```python
from build123d import *

# Parameters (mm, degrees)
SKETCH1_W            = 66.5
SKETCH1_H            = 64.5
BOSS_EXTRUDE1_DEPTH  = 25
SKETCH2_W            = 63.5
SKETCH2_H            = 61.5
CUT_EXTRUDE2_DEPTH   = 23.5
SKETCH9_W            = 10
SKETCH9_H            = 5
BOSS_EXTRUDE5_DEPTH  = 5
SKETCH14_R           = 1.5
CUT_EXTRUDE4_DEPTH   = 9
SKETCH17_W           = 10
SKETCH17_H           = 2.5
BOSS_EXTRUDE7_DEPTH  = 5
SKETCH18_R           = 1.5
CUT_EXTRUDE6_DEPTH   = 9
SKETCH19_R           = 1.5
BOSS_EXTRUDE9_DEPTH  = 8
SKETCH22_R           = 1.015
CUT_EXTRUDE7_DEPTH   = 7.5
SKETCH23_W           = 56
SKETCH23_H           = 20
BOSS_EXTRUDE12_DEPTH = 3
SKETCH26_W           = 42
SKETCH26_H           = 20
CUT_EXTRUDE9_DEPTH   = 3
CUT_EXTRUDE12_DEPTH  = 3
CUT_EXTRUDE13_DEPTH  = 3
SKETCH51_W           = 15
SKETCH51_H           = 8
CUT_EXTRUDE14_DEPTH  = 1.5


with BuildPart() as part:
    # Sketch1 → Boss-Extrude1 (new body)
    with BuildSketch(Plane.XY):
        Rectangle(SKETCH1_W, SKETCH1_H)
    extrude(amount=BOSS_EXTRUDE1_DEPTH)

    # Sketch2 → Cut-Extrude2 (cut)
    with BuildSketch(Plane.XY.offset(25)):
        Rectangle(SKETCH2_W, SKETCH2_H)
    extrude(amount=-CUT_EXTRUDE2_DEPTH, mode=Mode.SUBTRACT)

    # Sketch9 → Boss-Extrude5 (add)
    with BuildSketch(Plane.ZY.offset(33.25)):
        with Locations((20, 0)):
            Rectangle(SKETCH9_W, SKETCH9_H)
    extrude(amount=-BOSS_EXTRUDE5_DEPTH)

    # Sketch14 → Cut-Extrude4 (cut)
    with BuildSketch(Plane.XY.offset(25)):
        with Locations((-30.75, 0.228198866)):
            Circle(SKETCH14_R)
    extrude(amount=-CUT_EXTRUDE4_DEPTH, mode=Mode.SUBTRACT)

    # Sketch17 → Boss-Extrude7 (add)
    with BuildSketch(Plane(origin=(33.25, 0, 0), x_dir=(0, 0, -1), z_dir=(1, 0, 0))):
        with Locations((-20, 1.25)):
            Rectangle(SKETCH17_W, SKETCH17_H)
        with Locations((-20, -1.25)):
            Rectangle(SKETCH17_W, SKETCH17_H)
    extrude(amount=-BOSS_EXTRUDE7_DEPTH)

    # Sketch18 → Cut-Extrude6 (cut)
    with BuildSketch(Plane.XY.offset(25)):
        with Locations((30.75, 0)):
            Circle(SKETCH18_R)
    extrude(amount=-CUT_EXTRUDE6_DEPTH, mode=Mode.SUBTRACT)

    # Sketch19 → Boss-Extrude9 (add)
    with BuildSketch(Plane.XY.offset(1.5)):
        with Locations((-20.04, 29.09)):
            Circle(SKETCH19_R)
        with Locations(Location((30.04, 29.09, 0), (0, 0, 180))):
            Circle(SKETCH19_R)
        with Locations(Location((-20.04, -19.09, 0), (0, 0, 180))):
            Circle(SKETCH19_R)
        with Locations((30.04, -18.96)):
            Circle(SKETCH19_R)
    extrude(amount=BOSS_EXTRUDE9_DEPTH)

    # Sketch22 → Cut-Extrude7 (cut)
    with BuildSketch(Plane.XY.offset(9.5)):
        with Locations((-20.04, 29.09)):
            Circle(SKETCH22_R)
        with Locations((30.04, 29.049098521)):
            Circle(SKETCH22_R)
        with Locations((30.04, -18.96)):
            Circle(SKETCH22_R)
        with Locations((-20.04, -19.09)):
            Circle(SKETCH22_R)
    extrude(amount=-CUT_EXTRUDE7_DEPTH, mode=Mode.SUBTRACT)

    # Sketch23 → Boss-Extrude12 (add)
    with BuildSketch(Plane.XY.offset(1.5)):
        with Locations((3.75, 14.75)):
            Rectangle(SKETCH23_W, SKETCH23_H)
    extrude(amount=BOSS_EXTRUDE12_DEPTH)

    # Sketch26 → Cut-Extrude9 (cut)
    with BuildSketch(Plane.XY.offset(4.5)):
        with Locations((4.75, 14.75)):
            Rectangle(SKETCH26_W, SKETCH26_H)
    extrude(amount=-CUT_EXTRUDE9_DEPTH, mode=Mode.SUBTRACT)

    # Sketch45 → Cut-Extrude12 (cut)
    with BuildSketch(Plane(origin=(33.25, 0, 0), x_dir=(0, 0, -1), z_dir=(1, 0, 0))):
        Polygon((-9.814807173, 15.135540206), (-6.214807173, 15.135540206), (-6.214807173, 24.735863123), (-6.214807173, 25.135540206), (-9.814807173, 25.135540206), align=None)
        Polygon((-6.214807173, 4.436476389), (-6.214807173, 13.135540206), (-9.714807173, 13.135540206), (-9.714807173, 3.135540206), (-6.214807173, 3.135540206), align=None)
    extrude(amount=-CUT_EXTRUDE12_DEPTH, mode=Mode.SUBTRACT)

    # Sketch46 → Cut-Extrude13 (cut)
    with BuildSketch(Plane(origin=(0, 32.25, 0), x_dir=(1, 0, 0), z_dir=(0, 1, 0))):
        Polygon((-11.263140916, -11.9), (-11.75, -11.9), (-11.75, -21.9), (-1.75, -21.9), (-1.75, -11.9), align=None)
    extrude(amount=-CUT_EXTRUDE13_DEPTH, mode=Mode.SUBTRACT)

    # Sketch51 → Cut-Extrude14 (cut)
    with BuildSketch(Plane(origin=(0, 32.25, 0), x_dir=(1, 0, 0), z_dir=(0, 1, 0))):
        with Locations((16.75, -15.9)):
            Rectangle(SKETCH51_W, SKETCH51_H)
    extrude(amount=-CUT_EXTRUDE14_DEPTH, mode=Mode.SUBTRACT)


solid = part.part
```
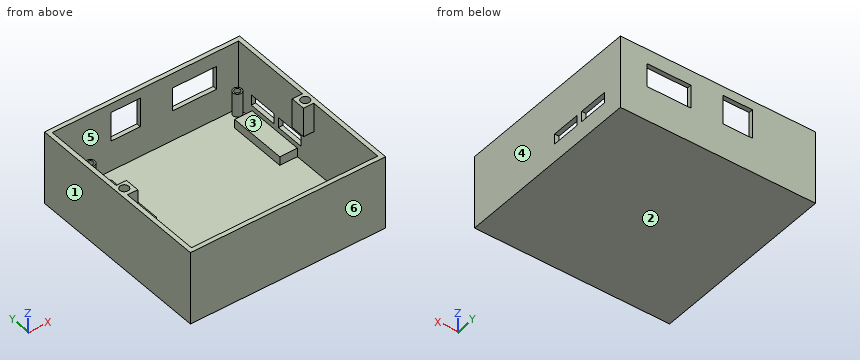
Input: part model. Units: mm. Frame: model coordinates. Face numbers are marked on the shaded views. A direction names the side the tool comes from. Round coordinates to 2 decimals unless told otherwise and drop trailing zeros. Loops run counter-clockwise (first coordinate to the right, second up) from the corner with the lowest first, then second, coordinate; pieces in that order, holes last. Notation, with made-up numbers: (-15, 85.5) - (15, 85.5) arc R24 cw to (15, 101.5) - close; hole circle Ø11 at (32.5, 70.5). An arc over 180 degrees is marked (long way). One line per item, written item: value. Start each with the question number.
(1) Draft query along X for the marked faces 1, 2, 3 and 4. Return one class per face: +X half, -X half, draft (parallel to the pull), parting line (faces both ways), or undercut.
(2) Access query for the marked faces 5 and 6. Directions: +Z, -Z, +X, -X, +Y, -Y. A direction counts if a zero-diameter tool reaches every point of the face in a straight line with its end or side. Return the directions, or none.
(3) Section D-D, the plane z = 8. Count the separate pieces of the cut face and the enclosed holes in it, plus the area to 3 significant figures.
(4) Section C-C, the plane y = 8. Return loops of the section in (x, z), plus the area to 3 significant figures.
(5) Contact query for flat-ended pins moving along their axis: P1, Ø4, axis at x = 0, y = -10, coming from the -Z side; P2, Ø6, axis at x = 13.5, y = -5.5, coming from the +Z side; P3, Ø0.9, axis at x = 31, y = 0, coming from the +Z side; P4, Ø8, axis at x = 25, y = 16, coming from the +Z side. Output: stop coordinate, or through.
(6) Ray query, line 1 (Y direction, x = -29, z = 21.25); line 2 (Y direction, x = -20.04, z = 4.75) (3 decimals); line 3 (Y direction, x = 30.04, z = 6.5) (3 decimals). Return the intervals inside material, ascending. Write a range as [from, to].
(7) Section B-B, the plane x = -10. Return loops of the section in (y, z), plus the area to 3 significant figures.
(8) Section A-A, the plane z = 17.5. Return loops of the section in (x, y).
Results below:
1. face 1: -X half
1. face 2: draft
1. face 3: undercut
1. face 4: +X half
2. face 5: +Z
2. face 6: +Z, -Z, +X, -X, -Y
3. separate pieces: 6
3. enclosed holes: 4
3. area: 369 mm^2
4. outline: (-33.25, 0) - (33.25, 0) - (33.25, 6.21) - (31.75, 6.21) - (31.75, 4.5) - (25.75, 4.5) - (25.75, 1.5) - (-16.25, 1.5) - (-16.25, 4.5) - (-24.25, 4.5) - (-24.25, 1.5) - (-31.75, 1.5) - (-31.75, 25) - (-33.25, 25) - close; (31.75, 9.71) - (33.25, 9.71) - (33.25, 25) - (31.75, 25) - close
4. area: 207 mm^2
5. P1: z = 0
5. P2: z = 1.5
5. P3: z = 16
5. P4: z = 4.5
6. line 1: [-32.25, -30.75], [-2.5, 2.5], [30.75, 32.25]
6. line 2: [-32.25, -30.75], [-20.59, -20.105], [-18.075, -17.59], [27.59, 28.075], [30.105, 30.59], [30.75, 32.25]
6. line 3: [-32.25, -30.75], [-20.46, -19.975], [-17.945, -17.46], [27.59, 28.034], [30.064, 30.59], [30.75, 32.25]
7. outline: (-32.25, 0) - (32.25, 0) - (32.25, 11.9) - (30.75, 11.9) - (30.75, 1.5) - (-30.75, 1.5) - (-30.75, 25) - (-32.25, 25) - close; (30.75, 21.9) - (32.25, 21.9) - (32.25, 25) - (30.75, 25) - close
7. area: 152 mm^2
8. outline: (-33.25, -32.25) - (33.25, -32.25) - (33.25, 32.25) - (24.25, 32.25) - (24.25, 30.75) - (31.75, 30.75) - (31.75, 2.5) - (28.25, 2.5) - (28.25, -2.5) - (31.75, -2.5) - (31.75, -30.75) - (-31.75, -30.75) - (-31.75, -2.5) - (-28.25, -2.5) - (-28.25, 2.5) - (-31.75, 2.5) - (-31.75, 30.75) - (-11.75, 30.75) - (-11.75, 32.25) - (-33.25, 32.25) - close; (-1.75, 30.75) - (9.25, 30.75) - (9.25, 32.25) - (-1.75, 32.25) - close; hole circle Ø3 at (-30.75, 0.23); hole circle Ø3 at (30.75, 0)
